from build123d import *

# Parameters (mm, degrees)
F0_R     = 5
F1_DEPTH = 3.2
F0_R_2   = 1.15
F2_DEPTH = 2
F3_DEPTH = 5
F4_SIZE  = 2
F5_ANGLE = 180


with BuildPart() as f1:
    # F0 (on Top) → F1 (new body)
    with BuildSketch(Plane.XY):
        with BuildLine():
            ThreePointArc((6.873864, -3), (7.341797, -1.532322), (7.5, 0))
            ThreePointArc((7.5, 0), (7.341797, 1.532322), (6.873864, 3))
            ThreePointArc((6.873864, 3), (0, 7.5), (-6.873864, 3))
            ThreePointArc((-6.873864, 3), (-7.5, 0), (-6.873864, -3))
            ThreePointArc((-6.873864, -3), (0, -7.5), (6.873864, -3))
        make_face()
        Circle(F0_R, mode=Mode.SUBTRACT)
    extrude(amount=F1_DEPTH)

    # F0 (on Top) → F2 (join)
    with BuildSketch(Plane.XY):
        with BuildLine():
            ThreePointArc((-6.873864, 3), (0, 7.5), (6.873864, 3))
            Line((6.873864, 3), (12.5, 3))
            Line((12.5, 3), (12.5, 12.5))
            Line((12.5, 12.5), (-12.5, 12.5))
            Line((-12.5, 12.5), (-12.5, 3))
            Line((-12.5, 3), (-6.873864, 3))
        make_face()
        with Locations((-10.5, 10.5)):
            Circle(F0_R_2, mode=Mode.SUBTRACT)
        with Locations((10.5, 10.5)):
            Circle(F0_R_2, mode=Mode.SUBTRACT)
        with BuildLine():
            Line((12.5, -3), (6.873864, -3))
            ThreePointArc((6.873864, -3), (0, -7.5), (-6.873864, -3))
            Line((-6.873864, -3), (-12.5, -3))
            Line((-12.5, -3), (-12.5, -12.5))
            Line((-12.5, -12.5), (12.5, -12.5))
            Line((12.5, -12.5), (12.5, -3))
        make_face()
        with Locations((-10.5, -10.5)):
            Circle(F0_R_2, mode=Mode.SUBTRACT)
        with Locations((10.5, -10.5)):
            Circle(F0_R_2, mode=Mode.SUBTRACT)
    extrude(amount=F2_DEPTH)

    # F0 (on Top) → F3 (join)
    with BuildSketch(Plane.XY):
        with BuildLine():
            ThreePointArc((-6.873864, -3), (-7.5, 0), (-6.873864, 3))
            Line((-6.873864, 3), (-12.5, 3))
            Line((-12.5, 3), (-12.5, -3))
            Line((-12.5, -3), (-6.873864, -3))
        make_face()
        with BuildLine():
            ThreePointArc((6.873864, 3), (7.341797, 1.532322), (7.5, 0))
            ThreePointArc((7.5, 0), (7.341797, -1.532322), (6.873864, -3))
            Line((6.873864, -3), (12.5, -3))
            Line((12.5, -3), (12.5, 3))
            Line((12.5, 3), (6.873864, 3))
        make_face()
    extrude(amount=F3_DEPTH)

    # F4
    f4_edges = [f1.edges().sort_by_distance(p)[0] for p in [
        (-5, 0, 0),
    ]]
    chamfer(f4_edges, length=F4_SIZE)


with BuildPart() as f1_1:
    # F5: moved
    add(f1.part.rotate(Axis((9.686932, -3, 5), (1, 0, 0)), F5_ANGLE))


solid = f1_1.part
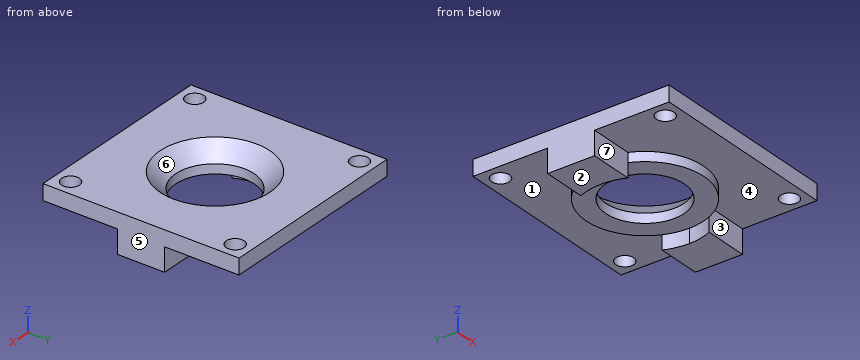
Could you check a few things on this model? Use its own coordinates, in mm. Face numbers are marked on the shaded views. A direction names the side the tool comes from. Give positions to 0.01 mm unless a question says otherwise; leave off trailing zeros. Order: outer loops, then holes, each group sorted by start corner. A loop starts at its lowest first (then second) coordinate and runs counter-clockwise, first axis right, second up. Notation, with made-up numbers: (3, -10.5) - (17, -10.5) arc R26 ccw to (17, 12.5) - close; hole circle Ø6 at (4, -4). An arc over 180 degrees is marked (long way). Return JSON: item names as keys, results as strings. Group by question number.
Q1. Suppose I cut it at B-B, the plane x = -10.5. Please give me the cut outline in (y, z), and give its area (3 significant figures).
Q2. Which directions (+Z, -Z, +X, -X, +Y, -Y) give clear straight access to the entire face, cutting with the end or side of a thin tool? Please do the marked faces 1, 2, 3 and 4.
Q3. Please list where these lines run through material, in increasing order: line 1 along Y through (x, z) = (10.5, 9.05); line 2 along X through (y, z) = (4.5, 9.2); line 3 along Y through (x, z) = (11, 8.4). Write a range as [from, to].
Q4. Suppose I cut it at D-D, the plane z = 9. Please give me the cut outline in (x, y), and give its area (3 significant figures).
Q5. Thinking about a two-plate mould opening in Y: for the marked faces 5, 6 and 7, which applies, pulls with the +Y half, pulls with the -Y half, needs draft (parallel to the pull), parting line crosses it, or undercut?
Q6. Will these pins go through, and if not, where does the flat tip stop? pin 1 Ø7.5 at (x, y) = (-2, -9) entering from -Z; pin 2 Ø2.5 at (x, z) = (11, 6) entering from -Y; pin 3 Ø2.5 at (x, y) = (-10.5, -16.5) entering from -Z.
Q7. Suppose I cut it at A-A, the plane z = 6.1. Please give me the cut outline in (x, y).
Q8. Suppose I cut it at C-C, the plane x = 0. Please give me the cut outline in (y, z).
Resolved:
{
 "1": {"outline": "(-18.5, 8) - (-17.65, 8) - (-17.65, 10) - (-18.5, 10) - close; (-15.35, 8) - (-9, 8) - (-9, 5) - (-3, 5) - (-3, 8) - (3.35, 8) - (3.35, 10) - (-15.35, 10) - close; (5.65, 8) - (6.5, 8) - (6.5, 10) - (5.65, 10) - close", "area": "58.8 mm2"},
 "2": {"face 1": "-Z, +Y", "face 2": "-Z, +X, -X, +Y, -Y", "face 3": "-Z, +X, -Y", "face 4": "-Z, -Y"},
 "3": {"line 1": "y = [-18.5, -17.65], [-15.35, 3.35], [5.65, 6.5]", "line 2": "x = [-12.5, -11.65], [-9.35, 9.35], [11.65, 12.5]", "line 3": "y = [-18.5, -17.54], [-15.46, 3.46], [5.54, 6.5]"},
 "4": {"outline": "(-12.5, -18.5) - (12.5, -18.5) - (12.5, 6.5) - (-12.5, 6.5) - close; hole circle Ø2.3 at (-10.5, -16.5); hole circle Ø2.3 at (-10.5, 4.5); hole circle Ø12 at (0, -6); hole circle Ø2.3 at (10.5, -16.5); hole circle Ø2.3 at (10.5, 4.5)", "area": "495 mm2"},
 "5": {"face 5": "needs draft", "face 6": "undercut", "face 7": "pulls with the -Y half"},
 "6": {"pin 1": "stops at z = 6.8", "pin 2": "stops at y = -9", "pin 3": "stops at z = 8"},
 "7": {"outline": "(-12.5, -9) - (-6.87, -9) arc R7.5 cw to (-6.87, -3) - (-12.5, -3) - close; (6.87, -9) - (12.5, -9) - (12.5, -3) - (6.87, -3) arc R7.5 cw to (7.5, -6) arc R7.5 cw to start"},
 "8": {"outline": "(-18.5, 8) - (-13.5, 8) - (-13.5, 6.8) - (-11, 6.8) - (-11, 8) - (-13, 10) - (-18.5, 10) - close; (-1, 6.8) - (1.5, 6.8) - (1.5, 8) - (6.5, 8) - (6.5, 10) - (1, 10) - (-1, 8) - close"}
}
